```python
from build123d import *

# Parameters (mm, degrees)
BOSS_EXTRUDE1_DEPTH     = 41.5
SKETCH3_W               = 8
SKETCH3_H               = 15
SKETCH3_W_2             = 3
SKETCH3_H_2             = 10
BOSS_EXTRUDE2_DEPTH     = 8
SKETCH3_3_W             = 16
SKETCH3_3_H             = 9
SKETCH3_3_W_2           = 10
SKETCH3_3_H_2           = 3
BOSS_EXTRUDE3_DEPTH     = 3
CUT_EXTRUDE1_DEPTH      = 104.688234627
CUT_EXTRUDE1_DEPTH_BACK = 83
SKETCH4_W               = 5
SKETCH4_H               = 3


with BuildPart() as part:
    # Sketch2 → Boss-Extrude1 (new, symmetric)
    with BuildSketch(Plane(origin=(0, 0, 0), x_dir=(0, 0, -1), z_dir=(1, 0, 0))):
        Polygon((-28.5, 8), (28.5, 8), (28.5, 20), (36.5, 20), (36.5, 0), (-36.5, 0), (-36.5, 20), (-28.5, 20), align=None)
    extrude(amount=BOSS_EXTRUDE1_DEPTH, both=True)

    # Sketch3 → Boss-Extrude2 (add)
    # profile 1 of 2: a face of its own
    with BuildSketch(Plane(origin=(0, 0, 0), x_dir=(1, 0, 0), z_dir=(0, 1, 0))):
        with Locations((-45.5, -29)):
            Rectangle(SKETCH3_W, SKETCH3_H)
        with Locations((-45.5, -29)):
            Rectangle(SKETCH3_W_2, SKETCH3_H_2, mode=Mode.SUBTRACT)
    # profile 2 of 2: a face of its own
    with BuildSketch(Plane(origin=(0, 0, 0), x_dir=(1, 0, 0), z_dir=(0, 1, 0))):
        with Locations((-45.5, 29)):
            Rectangle(SKETCH3_W, SKETCH3_H)
        with Locations((-45.5, 29)):
            Rectangle(SKETCH3_W_2, SKETCH3_H_2, mode=Mode.SUBTRACT)
    extrude(amount=BOSS_EXTRUDE2_DEPTH)

    # Sketch3<3> → Boss-Extrude3 (add)
    # profile 1 of 2: a face of its own
    with BuildSketch(Plane(origin=(0, 0, 0), x_dir=(1, 0, 0), z_dir=(0, 1, 0))):
        with Locations((0, -41)):
            Rectangle(SKETCH3_3_W, SKETCH3_3_H)
        with Locations((0, -41)):
            Rectangle(SKETCH3_3_W_2, SKETCH3_3_H_2, mode=Mode.SUBTRACT)
    # profile 2 of 2: a face of its own
    with BuildSketch(Plane(origin=(0, 0, 0), x_dir=(1, 0, 0), z_dir=(0, 1, 0))):
        with Locations((0, 41)):
            Rectangle(SKETCH3_3_W, SKETCH3_3_H)
        with Locations((0, 41)):
            Rectangle(SKETCH3_3_W_2, SKETCH3_3_H_2, mode=Mode.SUBTRACT)
    extrude(amount=BOSS_EXTRUDE3_DEPTH)

    # Sketch4 → Cut-Extrude1 (cut, two sides: drawn at the far end of the back side and taken through both)
    with BuildSketch(Plane(origin=(41.5, 0, 0), x_dir=(0, 0, -1), z_dir=(1, 0, 0)).offset(-CUT_EXTRUDE1_DEPTH_BACK)):
        with Locations((-34, 4.5)):
            Rectangle(SKETCH4_W, SKETCH4_H)
        with Locations((34, 4.5)):
            Rectangle(SKETCH4_W, SKETCH4_H)
    extrude(amount=CUT_EXTRUDE1_DEPTH + CUT_EXTRUDE1_DEPTH_BACK, mode=Mode.SUBTRACT)


solid = part.part
```
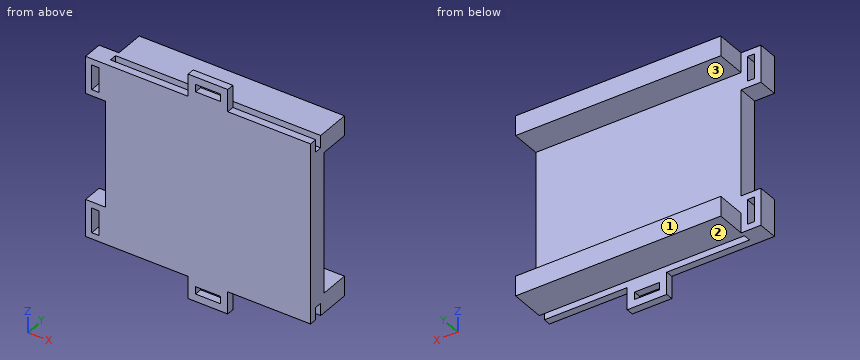
Can you work these out from the model? Positions are in its coordinate system, mm. Face numbers are marked on the shaded views. Coordinates: 2 decimals unless noted, no trailing zeros. Order: outer loops, then holes, each group sorted by start corner. A loop starts at its lowest first (then second) coordinate and runs counter-clockwise, first axis right, second up.
1. Thinking about a two-plate mould opening in Z: for the marked faces 1, 2 and 3, which applies, +Z half, -Z half, draft (parallel to the pull), parting line (faces both ways), or undercut?
2. If we section it at D-D (z = -3): Please give me the cut outline in (x, y).
3. I'm going to push flat-ended pins straight in: pin 1 (8 mm diameter, centred on x = -37, y = 12, fed in from -Z); pin 2 (6.5 mm diameter, centred on y = 14, z = 30.5, fed in from -X); pin 3 (5 mm diameter, centred on x = -14, z = -22.5, fed in from +Y). Where does each tip first touch, or does it pass through?
4. If we section it at C-C (x = 23): Please give me the cut outline in (y, z), then the cut area to 3 significant figures.
5. I need wall thicknesses on line 1 (Z direction, x = -23.5, y = 15); line 2 (X direction, y = 4.5, z = -26); line 3 (Y direction, x = 11, z = -35.5). Which ranges of each line are inside material? Lowest first, please.
6. If we section it at B-B (y = 17.5): Please give me the cut outline in (x, z).
7. If we section it at A-A (x = 1.5): Please give me the cut outline in (y, z), then the cut area to 3 significant figures.
Entries:
1. face 1: draft
1. face 2: -Z half
1. face 3: undercut
2. outline: (-41.5, 0) - (41.5, 0) - (41.5, 8) - (-41.5, 8) - close
3. pin 1: stops at z = -36.5
3. pin 2: stops at x = -41.5
3. pin 3: stops at y = 8
4. outline: (0, -36.5) - (3, -36.5) - (3, -31.5) - (6, -31.5) - (6, -36.5) - (20, -36.5) - (20, -28.5) - (8, -28.5) - (8, 28.5) - (20, 28.5) - (20, 36.5) - (6, 36.5) - (6, 31.5) - (3, 31.5) - (3, 36.5) - (0, 36.5) - close
4. area: 746 mm2
5. line 1: z = -36.5 to -28.5, 28.5 to 36.5
5. line 2: x = -49.5 to -47, -44 to 41.5
5. line 3: y = 0 to 3, 6 to 20
6. outline: (-41.5, -36.5) - (41.5, -36.5) - (41.5, -28.5) - (-41.5, -28.5) - close; (-41.5, 28.5) - (41.5, 28.5) - (41.5, 36.5) - (-41.5, 36.5) - close
7. outline: (0, -45.5) - (3, -45.5) - (3, -42.5) - (0, -42.5) - close; (0, -39.5) - (3, -39.5) - (3, -31.5) - (6, -31.5) - (6, -36.5) - (20, -36.5) - (20, -28.5) - (8, -28.5) - (8, 28.5) - (20, 28.5) - (20, 36.5) - (6, 36.5) - (6, 31.5) - (3, 31.5) - (3, 39.5) - (0, 39.5) - close; (0, 42.5) - (3, 42.5) - (3, 45.5) - (0, 45.5) - close
7. area: 782 mm2
